Can you work these out from the model? Positions are in its coordinate system, mm. A direction names the side the tool comes from. Give positions to 0.01 mm unless a question says otherwise; leave off trailing zeros. Write each loop counter-clockwise with the first axis right and the second up, starting at its lowest first coordinate (ties: lowest second). Pieces come first, ordered by that corner, then holes.
1. I'm going to push flat-ended pins straight in: pin 1 (4 mm diameter, centred on x = 1.32, z = -7.5, fed in from +Y); pin 2 (1 mm diameter, centred on x = -14.5, y = 12.5, fed in from +Z); pin 3 (4 mm diameter, centred on y = 35, z = -6.5, fed in from -X); pin 4 (8 mm diameter, centred on x = 20.5, y = 26, fed in from -Z). Where does each tip first touch, or does it pass through?
2. Suppose I cut it at B-B (y = 29). Please give me the cut outline in (x, z), and give its area (3 significant figures).
3. Suppose I cut it at C-C (z = 7.5). Please give me the cut outline in (x, y).
4. On a 3-axis mill with a long thin cutter (end or side, diameter ignored), from which of +Z, -Z, +X, -X, +Y, -Y can I reach the whole of each face in a straight line? I mean faces 5 (the flat face through (8.822, 35, -7)), 6 (the flat face through (4, 32.369, -7)), 7 (the flat face through (-22.678, 19, 7)), 8 (the flat face through (-6.178, 35, -7)). Say none if no direction works.
5. If I drill on probe 1 along X at (y, z) = (25.5, 6); probe 2 along Y at (x, z) = (15, 7.5); probe 3 along Y at (x, z) = (7, -6.25), over which ranges is the centre line in solid material (lowest first)?
6. Suppose I cut it at A-A (z = -7.5). Please give me the cut outline in (x, y).
7. Suppose I cut it at D-D (x = 5). Please give me the cut outline in (y, z).
8. Thinking about a two-plate mould opening in Y: for faces 1 (the flat face through (1, 32.369, 7)), 2 (the flat face through (1, 6.369, 7)), 3 (the cylindrical face through (10.326, 34.834, -1.426)), 4 (the flat face through (1, 1.369, 5)), which applies, pulls with the +Y half, pulls with the -Y half, needs draft (parallel to the pull), parting line crosses it, or undercut?
```python
from build123d import *

# Parameters (mm, degrees)
F0_W     = 58
F0_H     = 36
F0_W_2   = 48
F0_H_2   = 26
F1_DEPTH = 5
F2_DEPTH = 10
F3_W     = 15
F3_H     = 5
F4_DEPTH = 15
F5_R     = 2.5
F6_DEPTH = 25
F7_R     = 5


# Not quite as in the source:
# - a feature names something its author has since deleted; it is built from what else it names


with BuildPart() as f1:
    # F0 (on Top) → F1 (new body)
    with BuildSketch(Plane.XY):
        with Locations((1.3224579843, 19.3690634753)):
            Rectangle(F0_W, F0_H)
        with Locations((1.3224579843, 19.3690634753)):
            Rectangle(F0_W_2, F0_H_2, mode=Mode.SUBTRACT)
        with Locations((1.3224579843, 19.3690634753)):
            Rectangle(F0_W_2, F0_H_2)
    extrude(amount=F1_DEPTH)

    # F0 (on Top) → F2 (join)
    with BuildSketch(Plane.XY):
        with Locations((1.3224579843, 19.3690634753)):
            Rectangle(F0_W, F0_H)
        with Locations((1.3224579843, 19.3690634753)):
            Rectangle(F0_W_2, F0_H_2, mode=Mode.SUBTRACT)
    extrude(amount=F2_DEPTH)

    # F3 (on face) → F4 (join)
    with BuildSketch(Plane(origin=(0, 0, 0), x_dir=(1, 0, 0), z_dir=(0, 0, -1))):
        with Locations((1.3224579843, -34.8690634753)):
            Rectangle(F3_W, F3_H)
    extrude(amount=F4_DEPTH)

    # F5 (on face) → F6 (cut)
    with BuildSketch(Plane.XZ.offset(-32.3690634753)):
        with Locations((1.3224579843, -7.5)):
            Circle(F5_R)
    extrude(amount=-F6_DEPTH, mode=Mode.SUBTRACT)

    # F7
    f7_edges = [f1.edges().sort_by_distance(p)[0] for p in [
        (8.822458, 34.869063, -15),
        (-6.177542, 34.869063, -15),
        (8.822458, 34.869063, 0),
        (-6.177542, 34.869063, 0),
    ]]
    fillet(f7_edges, radius=F7_R)


solid = f1.part
```
Checks:
1. pin 1: passes through
1. pin 2: stops at z = 5
1. pin 3: stops at x = -6.2
1. pin 4: stops at z = 0
2. outline: (-27.68, 0) - (30.32, 0) - (30.32, 10) - (25.32, 10) - (25.32, 5) - (-22.68, 5) - (-22.68, 10) - (-27.68, 10) - close
2. area: 340 mm2
3. outline: (-27.68, 1.37) - (30.32, 1.37) - (30.32, 37.37) - (-27.68, 37.37) - close; hole (-22.68, 6.37) - (25.32, 6.37) - (25.32, 32.37) - (-22.68, 32.37) - close
4. face 5: -Z, +X, +Y, -Y
4. face 6: -Z, +X, -X, -Y
4. face 7: +Z
4. face 8: -Z, -X, +Y, -Y
5. probe 1: x = -27.68 to -22.68, 25.32 to 30.32
5. probe 2: y = 1.37 to 6.37, 32.37 to 37.37
5. probe 3: y = 32.37 to 37.37
6. outline: (-6.18, 32.37) - (-1.18, 32.37) - (-1.18, 37.37) - (-6.18, 37.37) - close; (3.82, 32.37) - (8.82, 32.37) - (8.82, 37.37) - (3.82, 37.37) - close
7. outline: (1.37, 0) - (32.37, 0) - (32.37, -14.86) - (37.37, -14.86) - (37.37, 10) - (32.37, 10) - (32.37, 5) - (6.37, 5) - (6.37, 10) - (1.37, 10) - close
8. face 1: undercut
8. face 2: undercut
8. face 3: needs draft
8. face 4: pulls with the -Y half
